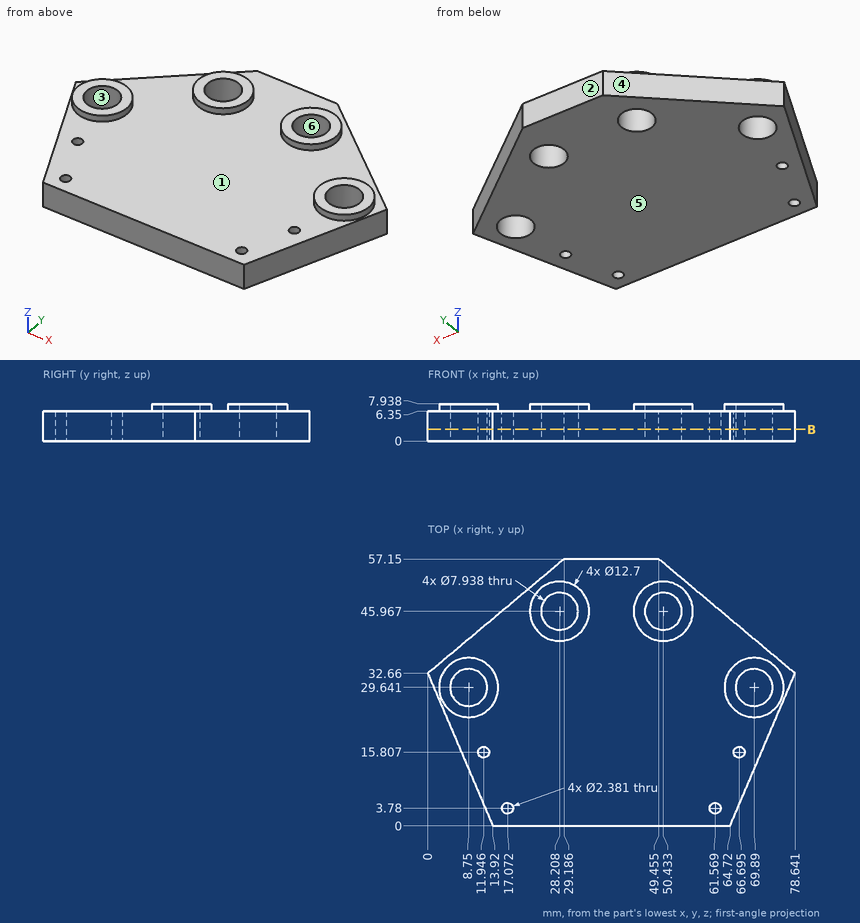
Study the drawing (mm; zero at the part's minimum x, y, z) and answer. A direction names the side the tool comes from. Coordinates: 2 decimals unless noted, no trailing zeros. Answer as a JSON object with one key per item and string values. Group by question number.
1. Which of the six approach directions +Z, -Z, +X, -X, +Y, -Y give full straight-line access (tool end or side, diameter ignored) to the marked faces 1 and 2?
2. A cutting plane is placed at B-B (z = 2.5). Give the number of separate pieces and of enclosed holes in the cut face, plus the area to 3 significant figures.
3. Each of these flat-tipped pins is pushed along its axis until it touches: P1, Ø6.5, axis at x = 28.21, y = 45.97, coming from the -Z side; P2, Ø1, axis at x = 10, z = 4.5, coming from the +Y side; P3, Ø1.5, axis at x = 22.5, y = 13.5, coming from the +Z side. Where does it stop, or does it pass through?
4. The mould has two halves that part along X. Classify the marked faces 3, 4, 5 and 6: +X half, -X half, draft (parallel to the pull), parting line (faces both ways), or undercut.
5. Consider L1, parallel to X at y = 31, z = 6 (1 decimal); L2, parallel to X at y = 43.5, z = 5.75 (1 decimal); L3, parallel to X at y = 27.5, z = 7.5. Determine where each line is inside the solid, lowest interval first. Write a range as [from, to].
Worked out:
{
 "1": {"face 1": "+Z", "face 2": "+Z, -Z, +X, -X, +Y"},
 "2": {"separate pieces": "1", "enclosed holes": "8", "area": "3,110 mm²"},
 "3": {"P1": "passes through", "P2": "stops at y = 41.47", "P3": "stops at z = 6.35"},
 "4": {"face 3": "undercut", "face 4": "-X half", "face 5": "draft", "face 6": "undercut"},
 "5": {"L1": "x = [0.7, 5], [12.5, 66.2], [73.6, 77.9]", "L2": "x = [12.9, 25.1], [31.3, 47.3], [53.5, 65.7]", "L3": "x = [2.77, 5.41], [12.09, 14.73], [63.91, 66.55], [73.23, 75.87]"}
}
